Autodesk Inventor part; units mm, degrees
ref_plane "РабПлоскость2" through (-53.0981, -74.1022, 20) normal (0, 0, -1) x (0.2079, 0.9781, 0)
ref_plane "YZ Plane" through (0, 0, 0) normal (1, 0, 0) x (0, 1, 0)
ref_plane "XZ Plane" through (0, 0, 0) normal (0, 1, 0) x (-1, 0, 0)
ref_plane "РабПлоскость1" through (0, 0, 0) normal (0, 0, 1) x (1, 0, 0)
sketch "Эскиз1" plane through (0, 0, 0) normal (0, 0, 1) x (1, 0, 0)
  circle A0 centre (-30.9426, -53.5039) radius 3 construction
  circle A1 centre (25.1804, -56.4452) radius 3 construction
  circle A2 centre (-25.1804, 56.4452) radius 3 construction
  circle A3 centre (30.9426, 53.5039) radius 3 construction
  circle A4 centre (-30.9426, -53.5039) radius 3.1
  circle A5 centre (25.1804, -56.4452) radius 3.1
  circle A6 centre (30.9426, 53.5039) radius 3.1
  circle A7 centre (-25.1804, 56.4452) radius 3.1
  line L0 (38.9316, 53.0852) -> (34.8315, -25.15)
  arc A8 (38.9316, 53.0852) -> (31.3613, 61.493) centre (30.9426, 53.5039) ccw
  line L1 (-24.7617, 64.4342) -> (31.3613, 61.493)
  arc A9 (-24.7617, 64.4342) -> (-33.1694, 56.8639) centre (-25.1804, 56.4452) ccw
  line L2 (-38.9316, -53.0852) -> (-33.1694, 56.8639)
  arc A10 (-38.9316, -53.0852) -> (-31.3613, -61.493) centre (-30.9426, -53.5039) ccw
  line L3 (-8.2929, -62.7019) -> (-31.3613, -61.493)
  line L4 (24.7617, -64.4342) -> (11.6797, -63.7486)
  arc A11 (24.7617, -64.4342) -> (33.1694, -56.8639) centre (25.1804, -56.4452) ccw
  line L5 (33.7848, -45.1226) -> (33.1694, -56.8639)
  line L6 (11.6797, -63.7486) -> (-8.2929, -62.7019)
  arc A12 (34.8315, -25.15) -> (33.7848, -45.1226) centre (35.2069, -35.1834) ccw
  circle A13 centre (35.2069, -35.1834) radius 4 construction
  arc A14 (34.989, -22.1448) -> (33.6273, -48.1278) centre (35.2069, -35.1834) ccw
  line L7 (31.9635, -22.5528) -> (35.7184, 49.0946)
  circle A15 centre (30.9426, 53.5039) radius 6.5
  circle A16 centre (-25.1804, 56.4452) radius 6.5
  circle A17 centre (25.1804, -56.4452) radius 6.5
  circle A18 centre (-30.9426, -53.5039) radius 6.5
  line L8 (27.0566, 58.7144) -> (-20.7711, 61.221)
  line L9 (30.3909, -52.5593) -> (30.661, -47.4059)
  line L10 (20.7711, -61.221) -> (-27.0566, -58.7144)
  line L11 (-35.7184, -49.0946) -> (-30.3909, 52.5593)
  point P0 (0, 0)
  dimension "d2" = 6.2
  dimension "d6" = 6
  dimension "d9" = 6.2
  dimension "d10" = 6.2
  dimension "d11" = 6.2
  dimension "d12" = 10.0404
  dimension "d13" = 13.0404
  dimension "d14" = 3
  dimension "d15" = 13
  dimension "d16" = 3
  dimension "d17" = 3
  dimension "d18" = 3
  dimension "d19" = 3
ref_plane "РабПлоскость2" through (-53.0981, -74.1022, 20) normal (0, 0, -1) x (0.2079, 0.9781, 0)
extrude "Выдавливание1" add sketch "Эскиз1" along normal up to surface (20 mm away) contours L0 A14 L7 A15 L8 A16 L11 A18 L10 A17 L9 L5 A11 L4 L6 L3 A10 L2 A9 L1 A8 | L0 A12 L5 A14 | A15 | A17 | A16 | A18
fillet "Сопряжение1" radius 2 10 edges at (20.7711, -61.221, 10) (30.3909, -52.5593, 10) (-35.7184, -49.0946, 10) (-27.0566, -58.7144, 10) (27.0566, 58.7144, 10) (35.7184, 49.0946, 10) (-20.7711, 61.221, 10) (-30.3909, 52.5593, 10) (31.9635, -22.5528, 10) (30.661, -47.4059, 10)
equation "\"d9\" = d2"
equation "\"d10\" = d2"
equation "\"d11\" = d2"
properties part number "Стойка" material "Сталь нержавеющая, 440C"
Source: CAD feature listing. Evaluate the final solid. Frame: model axes, mm. A direction names the side the tool comes from. Round coordinates to 2 decimals unless told otherwise and drop trailing zeros. Order: outer loops, then holes, each group sorted by start corner. A loop starts at its lowest first (then second) coordinate and runs counter-clockwise, first axis right, second up. Notation, with made-up numbers: (-11, 45) - (-6, 45) arc R32 cw to (-6, 76) - close; hole circle Ø8 at (88, 75.25). An arc over 180 degrees is marked (long way). Use a Markdown table: item, result. Add a question column.
1. Section query A-A (y = -35). Return the cut outline in (x, z), then the cut area to 3 significant figures.
2. Section query B-B (x = 14). Return the cut outline in (y, z), then the cut area to 3 significant figures.
3. Section query C-C (z = 12.75). Give the number of separate pieces and of enclosed holes in the cut face, then the cut area to 3 significant figures.
4. Mould query, pull axis Y, two halves, no side actions, for faces 3 (the flat face through (36.91, 14.52, 9.86)), 4 (the cylindrical face through (26.18, 49.08, 9.86)), 5 (the flat face through (2.907, 62.984, 9.86)). Classes: +Y half, -Y half, draft (parallel to the pull), parting line (faces both ways), or undercut.
5. First-contact query: pin 1 (1.5 mm diameter, centred on x = 6.5, z = 8, fed in from -Y); pin 2 (12 mm diameter, centred on y = -30, z = 12, fed in from -X); pin 3 (6 mm diameter, centred on x = 22, z = 11, fed in from -Y). Flat tips, straight axial feed; report the tip coordinate or a pass-through.
6. Set-up query: faces 1 (the flat face through (-35, 0, 20)), 2 (the flat face through (-33.09, 1.07, 9.86)). Return all of +Z, -Z, +X, -X, +Y, -Y with unobstructed straight access to the full face (end or side cutting, diameter ignored); none if empty.
7. Line query: probe 1 along Y at (x, z) = (31, 13); probe 2 along X at (y, z) = (55, 9.5); probe 3 along Y at (x, z) = (21.5, 1.25). Output: solid intervals per line, ascending.
Derived:
| question | item | result |
|---|---|---|
| 1 | outline | (-37.98, 0) - (-34.98, 0) - (-34.98, 20) - (-37.98, 20) - close; (22.17, 0) - (25.17, 0) - (25.17, 20) - (22.17, 20) - close |
| 1 | area | 120 mm2 |
| 2 | outline | (-63.87, 0) - (-60.87, 0) - (-60.87, 20) - (-63.87, 20) - close; (59.4, 0) - (62.4, 0) - (62.4, 20) - (59.4, 20) - close |
| 2 | area | 120 mm2 |
| 3 | separate pieces | 1 |
| 3 | enclosed holes | 5 |
| 3 | area | 1,490 mm2 |
| 4 | face 3 | -Y half |
| 4 | face 4 | undercut |
| 4 | face 5 | +Y half |
| 5 | pin 1 | y = -63.52 |
| 5 | pin 2 | x = -38.04 |
| 5 | pin 3 | y = -64.44 |
| 6 | face 1 | +Z, +X, -X, +Y, -Y |
| 6 | face 2 | +Z, -Z |
| 7 | probe 1 | -61.93 to -44.3, -26.07 to -22.81, 47 to 50.4, 56.6 to 61.51 |
| 7 | probe 2 | -33.27 to -27.92, -22.44 to -18.84, 24.62 to 28.23, 33.66 to 38.8 |
| 7 | probe 3 | -64.26 to -51.09, 59.01 to 62.01 |
